Could you check a few things on this model? Use its own coordinates, in mm. Face numbers are marked on the shaded views. A direction names the side the tool comes from. Give positions to 0.01 mm unless a question says otherwise; leave off trailing zeros. Loops run counter-clockwise (first coordinate to the right, second up) from the corner with the lowest first, then second, coordinate; pieces in that order, holes last. Notation, with made-up numbers: (2.25, 87.25) - (36.25, 87.25) arc R19 cw to (36.25, 94.25) - close; hole circle Ø9 at (89.5, 78). An arc over 180 degrees is marked (long way). Write each question's results on one line, items separated by ' | '. Start each with the question number.
1) On a 3-axis mill with a long thin cutter (end or side, diameter ignored), from which of +Z, -Z, +X, -X, +Y, -Y can I reach the whole of each face in a straight line? I mean the marked faces 1 and 2. Say none if no direction works.
2) If we mould it in two halves opening along Y, with no side actions, what happens to the marked faces 3, 4 and 5? For each: +Y half, -Y half, draft (parallel to the pull), parting line (faces both ways), or undercut.
3) I want a section at B-B, the plane x = 3. Write out the boundary of the cut face in (y, z), and give its area (3 significant figures).
4) I want a section at C-C, the plane y = 19.5. Write out the boundary of the cut face in (x, z).
5) I want a section at A-A, the plane y = 11.5. Write out the boundary of the cut face in (x, z), and give its area (3 significant figures).
6) If I drill on probe 1 along Z at (x, y) = (-11, -24.1); probe 2 along Y at (x, z) = (23.7, 27.5); probe 3 along Y at (x, z) = (24, 43), over which ranges is the centre line in solid material (lowest first)? Write a range as [from, to].
7) I'm going to push flat-ended pins straight in: pin 1 (1 mm diameter, centred on y = 4, z = 42, fed in from +X); pin 2 (5 mm diameter, centred on y = 11.5, z = 36.5, fed in from +X); pin 3 (3 mm diameter, centred on y = -12.5, z = 27.5, fed in from +X). Where does each tip first touch, or does it pass through?
8) I want a section at D-D, the plane z = 43. Write out the boundary of the cut face in (x, y).
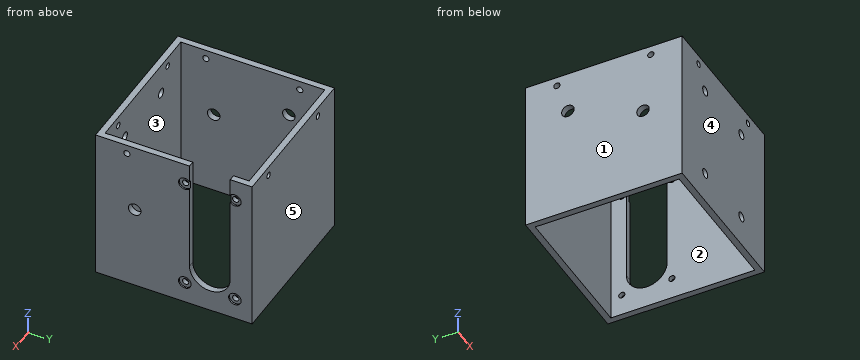
Autodesk Inventor part; units mm, degrees
ref_plane "YZ Plane" through (0, 0, 0) normal (1, 0, 0) x (0, 1, 0)
ref_plane "XZ Plane" through (0, 0, 0) normal (0, 1, 0) x (-1, 0, 0)
ref_plane "XY Plane" through (0, 0, 0) normal (0, 0, 1) x (1, 0, 0)
sketch "スケッチ1" plane through (0, 0, 0) normal (0, 0, 1) x (1, 0, 0)
  line L0 (-25, 25) -> (25, 25)
  line L1 (25, 25) -> (25, -25)
  line L2 (25, -25) -> (-25, -25)
  line L3 (-25, -25) -> (-25, 25)
  line L4 (-23, 23) -> (23, 23)
  line L5 (23, 23) -> (23, -23)
  line L6 (23, -23) -> (-23, -23)
  line L7 (-23, -23) -> (-23, 23)
  point P0 (0, 0)
  dimension "d0" = 50
  dimension "d1" = 50
  dimension "d4" = 25
  dimension "d5" = 25
  dimension "d6" = 46
  dimension "d7" = 2
  dimension "d8" = 46
  dimension "d9" = 2
extrude "押し出し1" add sketch "スケッチ1" along normal blind 50
sketch "スケッチ2" plane through (25, -25, 0) normal (1, 0, 0) x (0, 0, -1)
  line L0 (-50, 50) -> (-50, 0)
  line L1 (-50, 43) -> (-13.5, 43)
  line L2 (-13.5, 30) -> (-50, 30)
  line L3 (-50, 30) -> (-50, 43)
  arc A0 (-13.5, 30) -> (-13.5, 43) centre (-13.5, 36.5) ccw
  line L4 (0, 50) -> (-50, 50)
  point P0 (0, 25)
  point P1 (-11.7323, 30.245)
  dimension "d34" = 13
  dimension "d43" = 13
  dimension "d44" = 6.5
  dimension "d46" = 36.5
  dimension "d236" = 7
extrude "押し出し2" cut sketch "スケッチ2" against normal blind 30.5
sketch "スケッチ3" plane through (25, -25, 0) normal (1, 0, 0) x (0, 0, -1)
  arc A0 (-13.5, 30) -> (-13.5, 43) centre (-13.5, 36.5) ccw
  line L0 (-13.5, 30) -> (-50, 30)
  circle A1 centre (-7, 44.5) radius 1
  circle A2 centre (-43, 44.5) radius 1
  circle A3 centre (-43, 28.5) radius 1
  circle A4 centre (-7, 28.5) radius 1
  point P0 (0, 25)
  dimension "d47" = 8
  dimension "d48" = 8
  dimension "d49" = 16
  dimension "d50" = 1.5
  dimension "d51" = 36
  dimension "d52" = 36
  dimension "d53" = 6.5
  dimension "d55" = 2
  dimension "d56" = 6.5
hole "穴1" at (25, 3.5, 43) at (25, 19.5, 7) at (25, 3.5, 7) at (25, 19.5, 43) direction (-1, 0, 0) diameter 2 depth 2 tip angle 118 counterbore diameter 4 counterbore depth 0.5
sketch "スケッチ11" plane through (25, -25, 0) normal (1, 0, 0) x (0, 0, -1)
  circle A0 centre (-36.5, 36.5) radius 1.5
  line L0 (-50, 50) -> (-50, 43)
  circle A1 centre (-27.5, 12.5) radius 1.5
  line L1 (0, 50) -> (0, 0)
  line L2 (0, 50) -> (-50, 50)
  point P0 (0, 25)
  dimension "d109" = 3
  dimension "d128" = 24
  dimension "d237" = 13.5
  dimension "d238" = 27.5
  dimension "d239" = 13.5
hole "穴6" at (25, -12.5, 27.5) at (25, 11.5, 36.5) direction (-1, 0, 0) diameter 4 end through all
sketch "スケッチ18" plane through (-25, -25, 0) normal (0, -1, 0) x (1, 0, 0)
  line L0 (50, 50) -> (0, 50)
  line L1 (50, 0) -> (0, 0)
  circle A0 centre (14, 40) radius 1.5
  circle A1 centre (36, 40) radius 1.5
  circle A2 centre (14, 10) radius 1.5
  circle A3 centre (36, 10) radius 1.5
  line L2 (0, 0) -> (0, 50)
  line L3 (50, 0) -> (50, 50)
  point P0 (49.5, 0)
  point P1 (49.5, 50)
  point P2 (25, 0)
  dimension "d240" = 10
  dimension "d241" = 10
  dimension "d242" = 10
  dimension "d243" = 10
  dimension "d248" = 3
  dimension "d267" = 22
  dimension "d268" = 22
  dimension "d269" = 14
  dimension "d270" = 14
hole "穴13" at (-11, -25, 40) at (-11, -25, 10) at (11, -25, 40) at (11, -25, 10) direction (0, 1, 0) diameter 3 depth 2 tip angle 118
thread "ねじ13"
thread "ねじ14"
thread "ねじ15"
thread "ねじ16"
sketch "スケッチ19" plane through (-25, -25, 0) normal (-1, 0, 0) x (0, 0, 1)
  line L0 (50, 0) -> (50, 50)
  line L1 (0, 50) -> (50, 50)
  circle A0 centre (47, 40) radius 1.1
  circle A1 centre (47, 10) radius 1.1
  point P0 (0, 25)
  dimension "d271" = 2.2
  dimension "d273" = 30
  dimension "d274" = 10
  dimension "d275" = 3
  dimension "d276" = 3
hole "穴14" at (-25, 15, 47) at (-25, -15, 47) direction (1, 0, 0) diameter 2 end through all
sketch "スケッチ20" plane through (-25, -25, 0) normal (0, -1, 0) x (1, 0, 0)
  line L0 (50, 50) -> (0, 50)
  line L1 (0, 0) -> (0, 50)
  circle A0 centre (10, 47) radius 1.1
  circle A1 centre (40, 47) radius 1.1
  point P0 (25, 0)
  dimension "d284" = 2.2
  dimension "d287" = 10
  dimension "d288" = 30
  dimension "d289" = 3
  dimension "d290" = 3
hole "穴15" at (-15, -25, 47) at (15, -25, 47) direction (0, 1, 0) diameter 2 end through all
properties part number "04" material "アルミニウム 6061"
Answers:
1) face 1: +Z, -Z, -X, +Y, -Y | face 2: +Z, -Z
2) face 3: undercut | face 4: -Y half | face 5: +Y half
3) outline: (-25, 0) - (-23, 0) - (-23, 50) - (-25, 50) - close; (23, 0) - (25, 0) - (25, 50) - (23, 50) - close | area: 200 mm2
4) outline: (-25, 0) - (-23, 0) - (-23, 50) - (-25, 50) - close; (23, 0) - (25, 0) - (25, 5) - (24.5, 5) - (24.5, 6) - (23, 6) - close; (23, 8) - (24.5, 8) - (24.5, 9) - (25, 9) - (25, 41) - (24.5, 41) - (24.5, 42) - (23, 42) - close; (23, 44) - (24.5, 44) - (24.5, 45) - (25, 45) - (25, 50) - (23, 50) - close
5) outline: (-25, 0) - (-23, 0) - (-23, 34.5) - (-25, 34.5) - close; (-25, 38.5) - (-23, 38.5) - (-23, 50) - (-25, 50) - close; (23, 0) - (25, 0) - (25, 7) - (23, 7) - close | area: 106 mm2
6) probe 1: z = [0, 8.5], [11.5, 38.5], [41.5, 50] | probe 2: y = [-25, -14.5], [-10.5, 5], [18, 25] | probe 3: y = [-25, 2.5], [4.5, 5], [18, 18.5], [20.5, 25]
7) pin 1: stops at x = 24.5 | pin 2: stops at x = -23 | pin 3: passes through
8) outline: (-25, -25) - (25, -25) - (25, 1.5) - (24.5, 1.5) - (24.5, 2.5) - (23, 2.5) - (23, -23) - (-23, -23) - (-23, 23) - (23, 23) - (23, 20.5) - (24.5, 20.5) - (24.5, 21.5) - (25, 21.5) - (25, 25) - (-25, 25) - close; (23, 4.5) - (24.5, 4.5) - (24.5, 5) - (23, 5) - close; (23, 18) - (24.5, 18) - (24.5, 18.5) - (23, 18.5) - close
